Verification items for the finished model (mm, model axes). Face numbers are marked on the shaded views. Coordinates: 2 decimals unless noted, no trailing zeros. Order: outer loops, then holes, each group sorted by start corner. A loop starts at its lowest first (then second) coordinate and runs counter-clockwise, first axis right, second up. Notation, with made-up numbers: M 35.25,-30.75 L 84.25,-30.75 A29 ccw 84.25,-6.75 Z; hole C 40.5,26 d5. An arc over 180 degrees is marked long. Write item = value, one per line.
```python
from build123d import *

# Parameters (mm, degrees)
F2_R     = 5.08
F3_SIZE  = 5.08
F4_R     = 5.881856
F5_DEPTH = 6.351


with BuildPart() as f1:
    # F0 (on Front) → F1 (revolve)
    with BuildSketch(Plane.XZ):
        Polygon((-55.446185, 0), (0, 0), (0, 6.35), (-49.934152, 6.35), (-65.576335, 116.510788), (-71.863271, 115.61808), align=None)
    revolve(axis=Axis((0, 0, 3.175), (0, 0, -1)))

    # F2
    f2_edges = [f1.edges().sort_by_distance(p)[0] for p in [
        (49.934152, 0, 6.35),
    ]]
    fillet(f2_edges, radius=F2_R)

    # F3
    f3_edges = [f1.edges().sort_by_distance(p)[0] for p in [
        (65.576335, 0, 116.510788),
    ]]
    chamfer(f3_edges, length=F3_SIZE)

    # F4 (on face) → F5 (cut, through all)
    with BuildSketch(Plane.XY.offset(6.35)):
        with Locations((-17.260052, 19.45248)):
            Circle(F4_R)
        with Locations((-25.476368, -5.221403)):
            Circle(F4_R)
        with Locations((-8.216316, -24.673883)):
            Circle(F4_R)
        with Locations((17.260052, -19.45248)):
            Circle(F4_R)
        with Locations((25.476368, 5.221403)):
            Circle(F4_R)
        with Locations((8.216316, 24.673883)):
            Circle(F4_R)
    extrude(amount=-F5_DEPTH, mode=Mode.SUBTRACT)


solid = f1.part
```
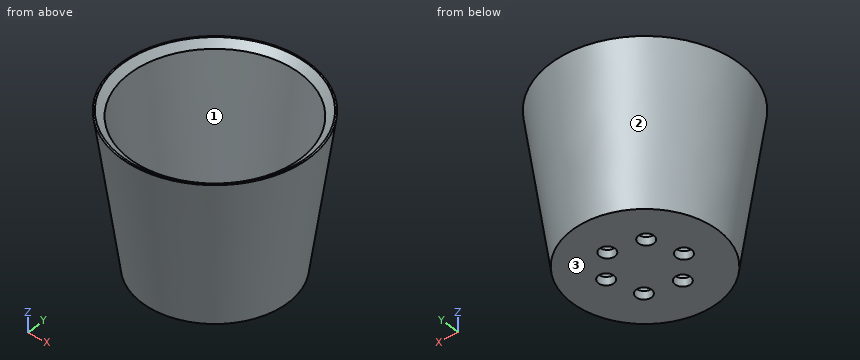
Item 1: Gauge pin test, flat ends, axial feed: pin 1 (1 mm diameter, centred on x = 21.5, z = 54.5, fed in from +Y); pin 2 (1.5 mm diameter, centred on x = -13, y = -33.5, fed in from -Z); pin 3 (1.5 mm diameter, centred on x = 46.5, y = -52, fed in from +Z); pin 4 (3 mm diameter, centred on x = 4.5, y = -40, fed in from +Z). Record the tip position at first contact, or that the pin passes through.
Report:
pin_1 = 59.61
pin_2 = 0
pin_3 = 115.72
pin_4 = 6.35
Item 2: Scan lines: L1, parallel to Z at x = 6.5, y = -14; L2, parallel to X at y = -20, z = 62; L3, parallel to X at y = -34, z = 66. Record each from-to range of solid material in increasing order. Write a range as from..to.
Report:
L1 = 0..6.35
L2 = -61.06..-54.27, 54.27..61.06
L3 = -55.18..-47.49, 47.49..55.18
Item 3: Release check for a two-part mould opening along Y. For the marked faces 1, 2 and 3 record: pulls with the +Y half, pulls with the -Y half, needs draft (parallel to the pull), parting line crosses it, or undercut.
Report:
face_1 = undercut
face_2 = parting line crosses it
face_3 = needs draft
Item 4: Sectioned sample at B-B, the plane y = 22. Give the number of separate pieces and of enclosed holes in the cut face, then the cut area to 3 significant figures.
Report:
separate_pieces = 3
enclosed_holes = 0
area = 2,010 mm^2
Item 5: Sectioned sample at A-A, the plane z = 92. Enter the section's corners in (x, y).
Report:
outline = C 0,0 d137.02; hole C 0,0 d124.19
Item 6: Sectioned sample at C-C, the plane z = 55. Enter the section's corners in (x, y), then the cut area to 3 significant figures.
Report:
outline = C 0,0 d126.51; hole C 0,0 d113.68
area = 2,420 mm^2
